from build123d import *

# Parameters (mm, degrees)
SKETCH_1_W          = 1000
SKETCH_1_H          = 100
EXTRUDE_1_DEPTH     = 5
HOLE_WIZARD_M24_1_D = 21


with BuildPart() as part:
    # 草图1 → 凸台-拉伸1 (new body, symmetric)
    with BuildSketch(Plane.XY):
        Rectangle(SKETCH_1_W, SKETCH_1_H)
    extrude(amount=EXTRUDE_1_DEPTH, both=True)

    # M24 螺纹孔1 (through all)
    with Locations(Plane.XY.offset(5)):
        with Locations((-450, 0), (450, 0)):
            Hole(HOLE_WIZARD_M24_1_D / 2)


solid = part.part
Geometry check sheet. Reference: the model listing, model coordinates, mm. Round coordinates to 2 decimals unless told otherwise and drop trailing zeros. Order: outer loops, then holes, each group sorted by start corner. A loop starts at its lowest first (then second) coordinate and runs counter-clockwise, first axis right, second up. Notation, with made-up numbers: (4.25, -16) -> (52.25, -16) arc R18 cw to (52.25, 11) -> close; hole circle Ø4 at (-7, -8). An arc over 180 degrees is marked (long way). Use one line per item in the form item = value.
1. Cross-section at A-A, the plane x = -450. Enter the section's corners in (y, z), plus the area to 3 significant figures.
Working result:
outline = (-50, -5) -> (-10.5, -5) -> (-10.5, 5) -> (-50, 5) -> close; (10.5, -5) -> (50, -5) -> (50, 5) -> (10.5, 5) -> close
area = 790 mm^2
2. Cross-section at B-B, the plane y = 0. Enter the section's corners in (x, z).
Working result:
outline = (-500, -5) -> (-460.5, -5) -> (-460.5, 5) -> (-500, 5) -> close; (-439.5, -5) -> (439.5, -5) -> (439.5, 5) -> (-439.5, 5) -> close; (460.5, -5) -> (500, -5) -> (500, 5) -> (460.5, 5) -> close
3. Scan lines: line 1 along Y through (x, z) = (450, 2); line 2 along X through (y, z) = (4.5, 2.5). Record each from-to range of solid material in increasing order. Write a range as from..to.
Working result:
line_1 = -50..-10.5, 10.5..50
line_2 = -500..-459.49, -440.51..440.51, 459.49..500
4. Mould release check, pull along Y, two halves, no side actions. Record for faces 1 (the face through (-7, 1, -5)), 2 (the face through (440.3, -4.02, -0.07)): pulls with the +Y half, pulls with the -Y half, needs draft (parallel to the pull), parting line crosses it, or undercut.
Working result:
face_1 = needs draft
face_2 = undercut
